```python
from build123d import *

# Parameters (mm, degrees)
ESQUISSE1_R             = 90
BOSS_EXTRU_1_DEPTH      = 10
ESQUISSE2_R             = 20
BOSS_EXTRU_2_DEPTH      = 93
ESQUISSE4_R             = 75
ESQUISSE4_R_2           = 72
ESQUISSE4_R_3           = 57
ESQUISSE4_R_4           = 54
ESQUISSE4_R_5           = 39
ESQUISSE4_R_6           = 36
ENL_V_MAT_EXTRU_1_DEPTH = 1
ENL_V_MAT_EXTRU_1_TAPER = 30
ESQUISSE5_R             = 20
ENL_V_MAT_EXTRU_2_DEPTH = 59
ESQUISSE6_R             = 4
BOSS_EXTRU_3_DEPTH      = 60


with BuildPart() as part:
    # Esquisse1 → Boss.-Extru.1 (new body)
    with BuildSketch(Plane(origin=(0, 0, 0), x_dir=(1, 0, 0), z_dir=(0, 1, 0))):
        Circle(ESQUISSE1_R)
    extrude(amount=BOSS_EXTRU_1_DEPTH)

    # Esquisse2 → Boss.-Extru.2 (add)
    with BuildSketch(Plane(origin=(0, 10, 0), x_dir=(1, 0, 0), z_dir=(0, 1, 0))):
        Circle(ESQUISSE2_R)
    extrude(amount=BOSS_EXTRU_2_DEPTH)

    # Esquisse4 → Enlèv. mat.-Extru.1 (cut)
    with BuildSketch(Plane.XZ):
        Circle(ESQUISSE4_R)
        Circle(ESQUISSE4_R_2, mode=Mode.SUBTRACT)
        Circle(ESQUISSE4_R_3)
        Circle(ESQUISSE4_R_4, mode=Mode.SUBTRACT)
        Circle(ESQUISSE4_R_5)
        Circle(ESQUISSE4_R_6, mode=Mode.SUBTRACT)
    extrude(amount=-ENL_V_MAT_EXTRU_1_DEPTH, taper=ENL_V_MAT_EXTRU_1_TAPER, mode=Mode.SUBTRACT)

    # Esquisse3 → Révolution2 (revolve)
    with BuildSketch(Plane(origin=(0, 0, 0), x_dir=(0, 0, -1), z_dir=(1, 0, 0))):
        with BuildLine():
            Line((-69.970754953, 105.094254483), (-74.970754953, 105.094254483))
            ThreePointArc((-74.970754953, 105.094254483), (-69.214189796, 86.164390325), (-53.893634743, 73.644071148))
            ThreePointArc((-53.893634743, 73.644071148), (-43.46448587, 66.535394214), (-36.80473888, 55.814004192))
            ThreePointArc((-36.80473888, 55.814004192), (-22.477497728, 37.096821257), (0, 30))
            Line((0, 30), (0, 35))
            ThreePointArc((0, 35), (-19.606403656, 41.190330611), (-32.103598704, 57.516731724))
            ThreePointArc((-32.103598704, 57.516731724), (-39.854721671, 69.995105534), (-51.992962878, 78.26872751))
            ThreePointArc((-51.992962878, 78.26872751), (-65.060675662, 88.947970814), (-69.970754953, 105.094254483))
        make_face()
    revolve(axis=Axis((0, 103, 0), (0, -1, 0)))

    # Esquisse5 → Enlèv. mat.-Extru.2 (cut)
    with BuildSketch(Plane(origin=(0, 103, 0), x_dir=(1, 0, 0), z_dir=(0, 1, 0))):
        Circle(ESQUISSE5_R)
    extrude(amount=-ENL_V_MAT_EXTRU_2_DEPTH, mode=Mode.SUBTRACT)

    # Esquisse6 → Boss.-Extru.3 (add)
    with BuildSketch(Plane(origin=(0, 44, 0), x_dir=(1, 0, 0), z_dir=(0, 1, 0))):
        Circle(ESQUISSE6_R)
    extrude(amount=BOSS_EXTRU_3_DEPTH)


solid = part.part
```
The listing builds one solid part. Answer for the finished solid, in the listing's coordinates (mm). A direction names the side the tool comes from. Coordinates: 2 decimals unless noted, no trailing zeros. Write each loop counter-clockwise with the first axis right and the second up, starting at its lowest first coordinate (ties: lowest second). Pieces come first, ordered by that corner, then holes. Notation, with made-up numbers: (83, 16) - (142, 16) arc R20 cw to (142, 40) - close; hole circle Ø8 at (69, 48.25). An arc over 180 degrees is marked (long way). Return JSON: item names as keys, results as strings. Group by question number.
Q1. Find the intervals of material crossed by line 1 along Y through (x, z) = (-63, -50); line 2 along X through (y, z) = (82, -3); line 3 along X through (y, z) = (42, 13), in increasing order. Write a range as [from, to].
Q2. The part is cut by section A-A on y = 65. Write down the section's boundary in (x, z).
Q3. For a pull along X with two mould halves and no side action, classify faces 4 (the flat face through (53, 0, -22)), 5 (the cylindrical face through (41.53, 4.93, 79.845)), 6 (the cylindrical face through (-4.336, 42.718, 19.524)) as +X half, -X half, draft (parallel to the pull), parting line (faces both ways), or undercut.
Q4. Which of the six approach directions +Z, -Z, +X, -X, +Y, -Y give full straight-line access (tool end or side, diameter ignored) to faces 1 (the flat face through (4.2, 44, -0.3)), 2 (the flat face through (50, 105.094, -50)), 3 (the flat face through (-46, 1, 30))?
Q5. The part is cut by section B-B on y = 27. Write down the section's boundary in (x, z).
Q6. Flat-ended cylindrical pins translate along their axes: pin 1 Ø8 at (x, z) = (-7.5, -28) entering from +Y; pin 2 Ø1.5 at (y, z) = (92.5, 30) entering from +X; pin 3 Ø10 at (x, z) = (33, 50) entering from +Y. Find the tip coordinate at first contact, or state that the pin passes through.
Evaluation:
{
 "1": {"line 1": "y = [0, 10]", "line 2": "x = [-65.86, -58.44], [-2.65, 2.65], [58.44, 65.86]", "line 3": "x = [-25.03, -16.13], [-15.2, 15.2], [16.13, 25.03]"},
 "2": {"outline": "circle Ø84.18 at (0, 0); circle Ø8 at (0, 0); hole circle Ø71.73 at (0, 0)"},
 "3": {"face 4": "draft", "face 5": "parting line", "face 6": "undercut"},
 "4": {"face 1": "+Y", "face 2": "+Z, -Z, +X, -X, +Y", "face 3": "-Y"},
 "5": {"outline": "circle Ø40 at (0, 0)"},
 "6": {"pin 1": "stops at y = 59.72", "pin 2": "stops at x = 66.52", "pin 3": "stops at y = 88.72"}
}
